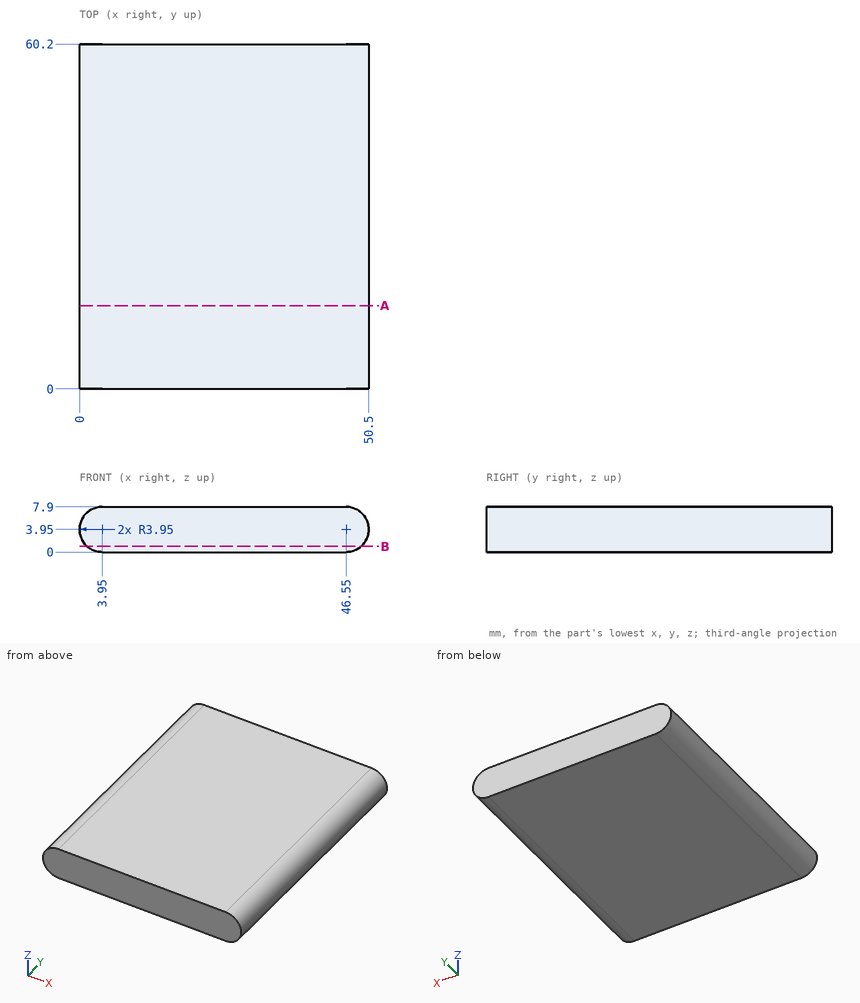
Geometry check sheet. Reference: drawing and pictorial views, mm from the part's lowest x, y, z. Round coordinates to 2 decimals unless told otherwise and drop trailing zeros. Order: outer loops, then holes, each group sorted by start corner. A loop starts at its lowest first (then second) coordinate and runs counter-clockwise, first axis right, second up. Notation, with made-up numbers: (51.25, 67.25) -> (61.25, 67.25) arc R6 cw to (61.25, 77.25) -> close; hole circle Ø9 at (10, 21). An arc over 180 degrees is marked (long way). One line per item, written item: value. Start each with the question number.
Q1. Cross-section at A-A (y = 14.5). Record the boundary of the cut face in (x, z), and give its area (3 significant figures).
Q2. Gauge pin test, flat end, axial feed: pin 1 Ø1.5 at (y, z) = (48, 1) entering from +X. Record the tip position at first contact, or that the pin passes through.
Q3. Cross-section at B-B (z = 1). Record the boundary of the cut face in (x, y), and give its area (3 significant figures).
Q4. Thickness scan on line 1 (X direction, y = 34.5, z = 3.75); line 2 (X direction, y = 15, z = 5). Record the ranges inside material, lowest first.
Completed:
1. outline: (3.95, 0) -> (46.55, 0) arc R3.95 ccw to (46.55, 7.9) -> (3.95, 7.9) arc R3.95 ccw to start
1. area: 386 mm²
2. pin 1: stops at x = 49.83
3. outline: (1.32, 0) -> (49.18, 0) -> (49.18, 60.2) -> (1.32, 60.2) -> close
3. area: 2,880 mm²
4. line 1: x = 0.01 to 50.49
4. line 2: x = 0.14 to 50.36
